from build123d import *

# Parameters (mm, degrees)
PAD_DEPTH       = 7
POCKET_DEPTH    = 5
SKETCH002_W     = 32
SKETCH002_H     = 3
PAD001_DEPTH    = 5
SKETCH003_W     = 10
SKETCH003_H     = 12
POCKET001_DEPTH = 2
PAD002_DEPTH    = 20
POCKET002_DEPTH = 5
SKETCH006_R     = 5
POCKET003_DEPTH = 7
PAD003_DEPTH    = 3
PAD004_DEPTH    = 40
CHAMFER_SIZE    = 5
CHAMFER001_SIZE = 5
CHAMFER002_SIZE = 3
CHAMFER003_SIZE = 1
CHAMFER004_SIZE = 1
SKETCH009_R     = 2.5
POCKET004_DEPTH = 39.001


with BuildPart() as part:
    # Sketch → Pad (new body)
    with BuildSketch(Plane.XY):
        Polygon((-23.5, 95), (23.5, 95), (23.5, 48), (20.5, 48), (20.5, 0), (-20.5, 0), (-20.5, 48), (-23.5, 48), align=None)
    extrude(amount=PAD_DEPTH)

    # Sketch001 (on Face9 of Pad) → Pocket (cut)
    with BuildSketch(Plane(origin=(0, 0, 0), x_dir=(1, 0, 0), z_dir=(0, 0, -1))):
        Polygon((-18.5, -2), (18.5, -2), (18.5, -50), (21.5, -50), (21.5, -93), (-21.5, -93), (-21.5, -50), (-18.5, -50), align=None)
    extrude(amount=-POCKET_DEPTH, mode=Mode.SUBTRACT)

    # Sketch002 (on Face5 of Pocket) → Pad001 (join)
    with BuildSketch(Plane.XY.offset(7)):
        with Locations((0, 44.5)):
            Rectangle(SKETCH002_W, SKETCH002_H)
        with Locations((0, 35.5)):
            Rectangle(SKETCH002_W, SKETCH002_H)
    extrude(amount=PAD001_DEPTH)

    # Sketch003 (on Face5 of Pad001) → Pocket001 (cut)
    with BuildSketch(Plane.XY.offset(7)):
        with Locations((-15.5, 81)):
            Rectangle(SKETCH003_W, SKETCH003_H)
    extrude(amount=-POCKET001_DEPTH, mode=Mode.SUBTRACT)

    # Sketch004 (on Face5 of Pocket001) → Pad002 (join)
    with BuildSketch(Plane.XY.offset(7)):
        Polygon((-9.5, 95), (15.5, 95), (15.5, 73), (13.5, 73), (13.5, 88), (-7.5, 88), (-7.5, 73), (-9.5, 73), align=None)
    extrude(amount=PAD002_DEPTH)

    # Sketch005 (on Face24 of Pad002) → Pocket002 (cut)
    with BuildSketch(Plane.YZ.offset(-7.5)):
        with BuildLine():
            ThreePointArc((87, 7), (81, 13), (75, 7))
            Line((75, 7), (87, 7))
        make_face()
    extrude(amount=-POCKET002_DEPTH, mode=Mode.SUBTRACT)

    # Sketch006 (on Face6 of Pad002) → Pocket003 (cut)
    with BuildSketch(Plane(origin=(0, 95, 0), x_dir=(-1, 0, 0), z_dir=(0, 1, 0))):
        with Locations((-3, 18)):
            Circle(SKETCH006_R)
    extrude(amount=-POCKET003_DEPTH, mode=Mode.SUBTRACT)

    # Sketch007 (on Face40 of Pocket003) → Pad003 (join)
    with BuildSketch(Plane.XY.offset(27)):
        Polygon((-9.5, 73), (-0.5, 73), (-0.5, 81), (6.5, 81), (6.5, 73), (15.5, 73), (15.5, 95), (-9.5, 95), align=None)
    extrude(amount=PAD003_DEPTH)

    # Sketch008 (on Face52 of Pad003) → Pad004 (join)
    with BuildSketch(Plane.XY.offset(30)):
        Polygon((-0.5, 73), (-0.5, 81), (6.5, 81), (6.5, 73), (9.5, 73), (9.5, 82), (2.5, 95), (-3.5, 82), (-3.5, 73), align=None)
    extrude(amount=PAD004_DEPTH)

    # Chamfer
    chamfer_edges = [part.edges().sort_by_distance(p)[0] for p in [
        (15.5, 95, 17),
    ]]
    chamfer(chamfer_edges, length=CHAMFER_SIZE)

    # Chamfer001
    chamfer001_edges = [part.edges().sort_by_distance(p)[0] for p in [
        (-9.5, 95, 17),
    ]]
    chamfer(chamfer001_edges, length=CHAMFER001_SIZE)

    # Chamfer002
    chamfer002_edges = [part.edges().sort_by_distance(p)[0] for p in [
        (6, 88.5, 70),
        (-0.5, 88.5, 70),
    ]]
    chamfer(chamfer002_edges, length=CHAMFER002_SIZE)

    # Chamfer003
    chamfer003_edges = [part.edges().sort_by_distance(p)[0] for p in [
        (0, 46, 12),
    ]]
    chamfer(chamfer003_edges, length=CHAMFER003_SIZE)

    # Chamfer004
    chamfer004_edges = [part.edges().sort_by_distance(p)[0] for p in [
        (0, 34, 12),
    ]]
    chamfer(chamfer004_edges, length=CHAMFER004_SIZE)

    # Sketch009 (on Face19 of Chamfer004) → Pocket004 (cut, through all)
    with BuildSketch(Plane.YZ.offset(15.5)):
        with Locations((78, 19)):
            Circle(SKETCH009_R)
    extrude(amount=-POCKET004_DEPTH, mode=Mode.SUBTRACT)


solid = part.part
Read the model definition and answer for the solid it produces. Units are mm, in the model's axes. A direction names the side the tool comes from. Round coordinates to 2 decimals unless told otherwise and drop trailing zeros. Write each loop counter-clockwise with the first axis right and the second up, starting at its lowest first coordinate (ties: lowest second). Pieces come first, ordered by that corner, then holes.
1. Straight lines are drawn through the part: L1, parallel to X at y = 85, z = 24.5; L2, parallel to Z at x = -6.5, y = 33; L3, parallel to Z at x = -8.1, y = 78. For each, find the intervals that lie inside material, in ascending order.
2. Which of the six approach directions +Z, -Z, +X, -X, +Y, -Y give full straight-line access (tool end or side, diameter ignored) to faces 4 (the face through (16, 35, 9)), 5 (the face through (15.5, 81, 18)), 6 (the face through (0, 93, 2))?
3. Given pin 1 Ø12 at (y, z) = (77, 45) entering from -X; pin 2 Ø4 at (y, z) = (28, 1.5) entering from +X; pin 3 Ø2 at (y, z) = (80, 19) entering from -X, each flat-ended and moving along its own axis, determine where each tip first touches the part or whether it passes through.
4. The part is cut by section D-D, the plane y = 31.5. Determine the outline of the cut face in (x, z), then the cut area to 3 significant figures.
5. The part is cut by section C-C, the plane z = 51. Determine the outline of the cut face in (x, y), then the cut area to 4 significant figures.
6. The part is cut by section A-A, the plane x = -13.5. Determine the outline of the cut face in (y, z).
7. Determine the mould class of faces 1 (the face through (4.08, 91.55, 13.12)), 2 (the face through (3, 81, 48)), 3 (the face through (-5, 84, 30)) for opening direction Z: pulls with the +Z half, pulls with the -Z half, needs draft (parallel to the pull), parting line crosses it, or undercut.
8. The part is cut by section B-B, the plane y = 85. Determine the outline of the cut face in (x, z), then the cut area to 3 significant figures.
Values:
1. L1: x = -9.5 to -7.5, 13.5 to 15.5
1. L2: z = 5 to 7
1. L3: z = 5 to 7, 12.2 to 16.5, 21.5 to 30
2. face 4: +Z, +X, +Y, -Y
2. face 5: +Z, +X, +Y
2. face 6: -Z
3. pin 1: stops at x = -3.5
3. pin 2: stops at x = 20.5
3. pin 3: stops at x = -9.5
4. outline: (-20.5, 0) - (-18.5, 0) - (-18.5, 5) - (18.5, 5) - (18.5, 0) - (20.5, 0) - (20.5, 7) - (-20.5, 7) - close
4. area: 102 mm2
5. outline: (-3.5, 73) - (-0.5, 73) - (-0.5, 81) - (6.5, 81) - (6.5, 73) - (9.5, 73) - (9.5, 82) - (2.5, 95) - (-3.5, 82) - close
5. area: 145.5 mm2
6. outline: (0, 0) - (2, 0) - (2, 5) - (75, 5) - (75, 7) - (46, 7) - (46, 11) - (45, 12) - (43, 12) - (43, 7) - (37, 7) - (37, 12) - (35, 12) - (34, 11) - (34, 7) - (0, 7) - close; (87, 5) - (93, 5) - (93, 0) - (95, 0) - (95, 7) - (87, 7) - close
7. face 1: undercut
7. face 2: needs draft
7. face 3: pulls with the +Z half
8. outline: (-23.5, 0) - (-21.5, 0) - (-21.5, 5) - (-20.5, 5) - (-20.5, 7) - (-23.5, 7) - close; (-10.5, 5) - (21.5, 5) - (21.5, 0) - (23.5, 0) - (23.5, 7) - (15.5, 7) - (15.5, 30) - (7.88, 30) - (7.88, 67) - (4.48, 70) - (1.19, 70) - (-2.12, 67) - (-2.12, 30) - (-9.5, 30) - (-9.5, 11.47) - (-7.5, 11.47) - (-7.5, 27) - (13.5, 27) - (13.5, 7) - (-10.5, 7) - close
8. area: 630 mm2
